from build123d import *

# Parameters (mm, degrees)
PAD_DEPTH            = 2
SKETCH001_R          = 2.5
SKETCH001_R_2        = 1
PAD003_DEPTH         = 11.5
SKETCH003_R          = 3
SKETCH003_R_2        = 1
PAD004_DEPTH         = 10.5
SKETCH006_R          = 2
SKETCH006_R_2        = 1
PAD007_DEPTH         = 1.25
PAD010_DEPTH         = 2
SKETCH008_W          = 10
SKETCH008_H          = 48
PAD009_DEPTH         = 10.5
SKETCH009_R          = 4.25
POCKET_DEPTH         = 47
PAD011_DEPTH         = 11.5
POCKET001_DEPTH      = 2
PAD012_DEPTH         = 11.5
POCKET002_DEPTH      = 2
SKETCH017_R          = 2
POCKET003_DEPTH      = 100
POCKET003_DEPTH_BACK = 100
POCKET004_DEPTH      = 3
POCKET005_DEPTH      = 3
POCKET006_DEPTH      = 9.5
PAD013_DEPTH         = 2
SKETCH023_R          = 28.5
SKETCH023_R_2        = 22.5
POCKET007_DEPTH      = 0.25


with BuildPart() as body:
    # Sketch → Pad (new body)
    with BuildSketch(Plane.XY):
        with BuildLine():
            Line((1.6382610688, 84.5131853633), (39.8652231068, 59.5943175186))
            ThreePointArc((40.9665622412, 57.0924822575), (40.788108314, 58.5072538624), (39.8652231068, 59.5943175186))
            Line((31.4665652521, -0.4074995185), (40.9665622412, 57.0924822575))
            Line((31.4665652521, -0.4074995185), (29.4686738682, -12.5))
            Line((-2.4238255474, -12.5), (29.4686738682, -12.5))
            Line((-2.999944227, 81.9817069741), (-2.4238255474, -12.5))
            ThreePointArc((1.6382610688, 84.5131853633), (-1.4372337891, 84.6333171164), (-2.999944227, 81.9817069741))
        make_face()
    extrude(amount=PAD_DEPTH)

    # Sketch001 (on Face9 of Pad) → Pad003 (join)
    with BuildSketch(Plane.XY.offset(2)):
        Circle(SKETCH001_R)
        Circle(SKETCH001_R_2, mode=Mode.SUBTRACT)
        with Locations((29, 0)):
            Circle(SKETCH001_R)
        with Locations((29, 0)):
            Circle(SKETCH001_R_2, mode=Mode.SUBTRACT)
        with Locations((38.5, 57.5)):
            Circle(SKETCH001_R)
        with Locations((38.5, 57.5)):
            Circle(SKETCH001_R_2, mode=Mode.SUBTRACT)
    extrude(amount=PAD003_DEPTH)

    # Sketch003 (on Face5 of Pad003) → Pad004 (join)
    with BuildSketch(Plane.XY.offset(2)):
        with Locations((0, 82)):
            Circle(SKETCH003_R)
        with Locations((0, 82)):
            Circle(SKETCH003_R_2, mode=Mode.SUBTRACT)
    extrude(amount=PAD004_DEPTH)

    # Sketch006 (on Face11 of Pad004) → Pad007 (join)
    with BuildSketch(Plane.XY.offset(12.5)):
        with Locations((0, 82)):
            Circle(SKETCH006_R)
        with Locations((0, 82)):
            Circle(SKETCH006_R_2, mode=Mode.SUBTRACT)
    extrude(amount=PAD007_DEPTH)

    # Sketch011 → Pad010 (join)
    with BuildSketch(Plane.XY):
        with BuildLine():
            Line((-7, 147.625513661), (3, 147.625513661))
            Line((3, 147.625513661), (3, 83.625513661))
            Line((1.6382610688, 84.5131853633), (3, 83.625513661))
            ThreePointArc((1.6382610688, 84.5131853633), (-1.4372359533, 84.6333159352), (-2.9999441969, 81.9817020431))
            Line((-2.9999441969, 81.9817020431), (-2.9694558253, 76.9817020431))
            Line((-7, 82), (-2.9694558253, 76.9817020431))
            Line((-7, 147.625513661), (-7, 82))
        make_face()
    extrude(amount=PAD010_DEPTH)

    # Sketch008 (on Face13 of Pad010) → Pad009 (join)
    with BuildSketch(Plane.XY.offset(2)):
        with Locations((-2, 123.625513661)):
            Rectangle(SKETCH008_W, SKETCH008_H)
    extrude(amount=PAD009_DEPTH)

    # Sketch009 (on Face22 of Pad009) → Pocket (cut)
    with BuildSketch(Plane.XZ.offset(-99.625513661)):
        with Locations((-2, 7.25)):
            Circle(SKETCH009_R)
    extrude(amount=-POCKET_DEPTH, mode=Mode.SUBTRACT)

    # Sketch012 (on Face4 of Pocket) → Pad011 (join)
    with BuildSketch(Plane.XY.offset(2)):
        with BuildLine():
            Line((4.5, 0), (2.5, 0))
            ThreePointArc((-2.4999535249, -0.0152438001), (0.0076219355, -2.4999883812), (2.5, 0))
            Line((-2.4238255474, -12.5), (-2.4999535249, -0.0152438001))
            Line((-2.4238255474, -12.5), (29.4686738682, -12.5))
            Line((29.4686738682, -12.5), (31.4665652521, -0.4074995185))
            ThreePointArc((26.4999999999, 0), (28.7955655729, -2.4916272926), (31.4665652521, -0.4074995185))
            Line((24.5, 0), (26.4999999999, 0))
            Line((24.5, 0), (24.5, -10.5))
            Line((4.5, -10.5), (24.5, -10.5))
            Line((4.5, 0), (4.5, -10.5))
        make_face()
    extrude(amount=PAD011_DEPTH)

    # Sketch013 (on Face16 of Pad011) → Pocket001 (cut)
    with BuildSketch(Plane(origin=(0, -10.5, 0), x_dir=(-1, 0, 0), z_dir=(0, 1, 0))):
        with BuildLine():
            ThreePointArc((-17, 11.25), (-20.5, 7.75), (-17, 4.25))
            Line((-17, 4.25), (-12, 4.25))
            ThreePointArc((-12, 4.25), (-8.5, 7.75), (-12, 11.25))
            Line((-17, 11.25), (-12, 11.25))
        make_face()
    extrude(amount=-POCKET001_DEPTH, mode=Mode.SUBTRACT)

    # Sketch014 → Pad012 (join)
    with BuildSketch(Plane.XY):
        Polygon((-7, 82), (-2.9694558253, 76.9817020431), (-2.4238255474, -12.5), (-7, -12.5), align=None)
        Polygon((40.9665622412, 57.0924822575), (29.4686738682, -12.5), (40.9665622412, -12.5), align=None)
    extrude(amount=PAD012_DEPTH)

    # Sketch016 (on DatumPlane) → Pocket002 (cut)
    with BuildSketch(Plane.YZ.offset(37.9665622412)):
        Polygon((51.6569219382, 6.75), (49.5784609691, 10.35), (45.4215390309, 10.35), (43.3430780618, 6.75), (45.4215390309, 3.15), (49.5784609691, 3.15), align=None)
    extrude(amount=POCKET002_DEPTH, mode=Mode.SUBTRACT)

    # Sketch017 (on DatumPlane) → Pocket003 (cut, two sides)
    with BuildSketch(Plane.YZ.offset(37.9665622412)) as pocket003_sk:
        with Locations((47.5, 6.75)):
            Circle(SKETCH017_R)
    extrude(amount=-POCKET003_DEPTH, mode=Mode.SUBTRACT)
    extrude(pocket003_sk.sketch, amount=POCKET003_DEPTH_BACK, mode=Mode.SUBTRACT)

    # Sketch018 (on Face13 of Pocket003) → Pocket004 (cut)
    with BuildSketch(Plane(origin=(-2.4999535243, -0.0152439024, 0), x_dir=(-0.006097561, 0.9999814097, 0), z_dir=(0.9999814097, 0.006097561, 0))):
        Polygon((51.6730491796, 6.75), (49.5945882105, 10.35), (45.4376662723, 10.35), (43.3592053032, 6.75), (45.4376662723, 3.15), (49.5945882105, 3.15), align=None)
    extrude(amount=-POCKET004_DEPTH, mode=Mode.SUBTRACT)

    # Sketch019 (on Face45 of Pocket004) → Pocket005 (cut)
    with BuildSketch(Plane.XY.offset(13.5)):
        with BuildLine():
            ThreePointArc((-2.4999535248, -0.0152438096), (0.0076219402, -2.4999883812), (2.5, 0))
            Line((2.5, 0), (4.5, 0))
            Line((4.5, 0), (4.5, -2.1794494718))
            ThreePointArc((-2.5263567378, 4.3148026181), (-3.3937655316, -3.671832719), (4.5, -2.1794494718))
            Line((-2.5263567378, 4.3148026181), (-2.4999535248, -0.0152438096))
        make_face()
        with BuildLine():
            ThreePointArc((24.5, -2.1794494718), (32.0941134062, -3.9276535272), (32.172405562, 3.8646918312))
            Line((31.4665660971, -0.4074944038), (32.172405562, 3.8646918312))
            ThreePointArc((26.4999999999, 0), (28.7955681562, -2.4916275046), (31.4665660971, -0.4074944038))
            Line((24.5, 0), (26.4999999999, 0))
            Line((24.5, -2.1794494718), (24.5, 0))
        make_face()
    extrude(amount=-POCKET005_DEPTH, mode=Mode.SUBTRACT)

    # Sketch021 (on Face38 of Pocket005) → Pocket006 (cut)
    with BuildSketch(Plane.XY.offset(11.5)):
        with BuildLine():
            ThreePointArc((-2.9694558253, 76.9817020431), (-4.3800712285, 76.387303242), (-4.9572235227, 74.9695441018))
            Line((-4.9572235227, 74.9695441018), (-4.8535649862, 57.9698601368))
            ThreePointArc((-4.8535649862, 57.9698601368), (-4.259166185, 56.5592447336), (-2.8414070448, 55.9820924394))
            Line((-2.8414070448, 55.9820924394), (-2.9694558253, 76.9817020431))
        make_face()
    extrude(amount=-POCKET006_DEPTH, mode=Mode.SUBTRACT)

    # Sketch022 → Pad013 (join)
    with BuildSketch(Plane.XY):
        with BuildLine():
            Line((40.9665622412, 12.9282777021), (40.9665622412, 57.0924822575))
            ThreePointArc((40.9665622412, 57.0924822575), (40.9384086484, 58.0515099848), (40.5511157715, 58.9293089561))
            ThreePointArc((40.9665622412, 12.9282777021), (51.4987766247, 36.0257883104), (40.5511157715, 58.9293089561))
        make_face()
    extrude(amount=PAD013_DEPTH)

    # Sketch023 (on Face7 of Pad013) → Pocket007 (cut)
    with BuildSketch(Plane(origin=(0, 0, 0), x_dir=(1, 0, 0), z_dir=(0, 0, -1))):
        with Locations((21.5, -35.7548620833)):
            Circle(SKETCH023_R)
        with Locations((21.5, -35.7548620833)):
            Circle(SKETCH023_R_2, mode=Mode.SUBTRACT)
    extrude(amount=-POCKET007_DEPTH, mode=Mode.SUBTRACT)


with BuildPart() as part_mirroring:
    # Part__Mirroring: instance of Body
    add(body.part.mirror(Plane(origin=(0, 0, 0), x_dir=(0, 1, 0), z_dir=(0, 0, 1))))


solid = part_mirroring.part
Check sheet for the modelled part. Datum: model origin and axes. Units: mm. A direction names the side the tool comes from. Round coordinates to 2 decimals unless told otherwise and drop trailing zeros. Loops run counter-clockwise (first coordinate to the right, second up) from the corner with the lowest first, then second, coordinate; pieces in that order, holes last. Notation, with made-up numbers: (-9.75, 55.5) - (28.25, 55.5) arc R15 ccw to (28.25, 74.5) - close; hole circle Ø9 at (-19, 49). An arc over 180 degrees is marked (long way). Answer as CSV lines item,"result". Start each with the question number.
Item 1: Section check B-B (y = 47). Count the separate pieces of the cut face and the enclosed holes in it, and give its area (3 significant figures).
Item 2: Release check for a two-part mould opening along X. For faces 6 (the cylindrical face through (8.5, -11.5, -7.7)), 7 (the flat face through (22, 36, 0)) record: +X half, -X half, draft (parallel to the pull), parting line (faces both ways), or undercut.
Item 3: Section check A-A (y = 116). Record the boundary of the cut face in (x, z).
Item 4: Section check D-D (y = 26). Record the boundary of the cut face in (x, z).
Item 5: Depth check by flat-ended pin: P1, Ø2, axis at y = 47, z = -5.5, coming from the -X side; P2, Ø3, axis at x = 0, y = 0, coming from the -Z side; P3, Ø24, axis at x = 17, y = 46.5, coming from the -Z side; P4, Ø0.6, axis at x = 3.5, z = -6.5, coming from the +Y side. Enter the tip coordinate at first touch or a pass-through.
Item 6: Scan lines: line 1 (Y direction, x = 0, z = -8.5); line 2 (Z direction, x = -2, y = 136); line 3 (Y direction, x = 2, z = -6.75). Record each from-to range of solid material in increasing order. Write a range as [from, to].
Item 7: Set-up check for faces 1 (the flat face through (42.5, 27.2, -0.25)), 2 (the flat face through (1, -1, -13.5)), 3 (the flat face through (-2, 124, -12.5)), 4 (the flat face through (39.967, 45, -7)), 5 (the flat face through (-5.013, 79.526, -6.684)): record each of +Z, -Z, +X, -X, +Y, -Y from which the full face is reachable in a straight line by a thin tool's end or side.
Item 8: Section check C-C (x = 22.5). Record the boundary of the cut face in (y, z), and give its area (3 significant figures).
Report:
1,separate pieces,"3"
1,enclosed holes,"0"
1,area,"130 mm2"
2,face 6,"undercut"
2,face 7,"draft"
3,outline,"(-7, -12.5) - (3, -12.5) - (3, 0) - (-7, 0) - close; hole circle Ø8.5 at (-2, -7.25)"
4,outline,"(-7, -11.5) - (-2.66, -11.5) - (-2.66, -2) - (35.83, -2) - (35.83, -11.5) - (40.97, -11.5) - (40.97, -2) - (49.87, -2) - (49.87, 0) - (48.28, 0) - (48.28, -0.25) - (41.78, -0.25) - (41.78, 0) - (1.22, 0) - (1.22, -0.25) - (-5.28, -0.25) - (-5.28, 0) - (-7, 0) - close"
5,P1,"stops at x = -7"
5,P2,"stops at z = -13.5"
5,P3,"stops at z = -2"
5,P4,"stops at y = 0"
6,line 1,"y = [-12.5, -1], [1, 2.5], [79, 81], [83, 85], [146.63, 147.63]"
6,line 2,"z = [-12.5, -11.5], [-3, 0]"
6,line 3,"y = [-12.5, 1.5], [79.76, 84.24], [146.63, 147.63]"
7,face 1,"+Z"
7,face 2,"-Z, +X, -X, -Y"
7,face 3,"-Z, +X, -X, +Y"
7,face 4,"none"
7,face 5,"-Z"
8,outline,"(-12.5, -13.5) - (-10.5, -13.5) - (-10.5, -2) - (70.91, -2) - (70.91, 0) - (64.24, 0) - (64.24, -0.25) - (58.23, -0.25) - (58.23, 0) - (13.28, 0) - (13.28, -0.25) - (7.27, -0.25) - (7.27, 0) - (-12.5, 0) - close"
8,area,"187 mm2"
